Geometry check sheet. Reference: the model listing, model coordinates, mm. A direction names the side the tool comes from. Give positions to 0.01 mm unless a question says otherwise; leave off trailing zeros. Write each loop counter-clockwise with the first axis right and the second up, starting at its lowest first coordinate (ties: lowest second). Pieces come first, ordered by that corner, then holes. Notation, with made-up numbers: (62.25, 7.25) - (102.25, 7.25) arc R10 ccw to (102.25, 25.25) - close; hole circle Ø1 at (51.5, 77). An arc over 180 degrees is marked (long way). Use a Markdown table: item, result.
```python
from build123d import *
from build123d.topology import SkipClean

# Parameters (mm, degrees)
CUT_EXTRUDE_1_REACH             = 16.541
CUT_EXTRUDE_1_DIRECTION_2_DEPTH = 10
PATTERN_CIRCULAR_1_COUNT        = 6
EXTRUDE_1_DEPTH                 = 1
PATTERN_CIRCULAR_2_COUNT        = 4


with BuildPart() as part:
    # Sketch 1 → Revolve 2 (revolve)
    with BuildSketch(Plane.XY, mode=Mode.PRIVATE) as revolve_2_sk:
        Polygon((-1.494617613, 7.636753237), (-8, 1.13137085), (-8.75, 1.13137085), (-8.75, 0.63137085), (-6.2372583, 0.63137085), (-0.363246763, 6.505382387), align=None)
    revolve(revolve_2_sk.sketch.rotate(Axis((0, 35.786073675, 0), (0, -1, 0)), 90), axis=Axis((0, 35.786073675, 0), (0, -1, 0)))

    # Sketch 2 → Cut-Extrude 1 (cut, up to next)
    with BuildSketch(Plane(origin=(0, 0, 0), x_dir=(1, 0, 0), z_dir=(0, 1, 0)), mode=Mode.PRIVATE) as cut_extrude_1_sk1:
        with BuildLine():
            Line((0, -0.1), (7.999374976, -0.1))
            ThreePointArc((7.999374976, -0.1), (8, 0), (7.999374976, 0.1))
            Line((7.999374976, 0.1), (0, 0.1))
            Line((0, 0.1), (0, -0.1))
        make_face()
    cut_extrude_1_tool1 = extrude(cut_extrude_1_sk1.sketch, amount=CUT_EXTRUDE_1_REACH, mode=Mode.PRIVATE) & part.part
    cut_extrude_1 = cut_extrude_1_tool1.solids().sort_by_distance((3.999896, 0, 0))[0]
    add(cut_extrude_1, mode=Mode.SUBTRACT)

    # Sketch 2 → Cut-Extrude 1 direction 2 (cut)
    with BuildSketch(Plane(origin=(0, 0, 0), x_dir=(1, 0, 0), z_dir=(0, 1, 0))):
        with BuildLine():
            Line((0, -0.1), (7.999374976, -0.1))
            ThreePointArc((7.999374976, -0.1), (8, 0), (7.999374976, 0.1))
            Line((7.999374976, 0.1), (0, 0.1))
            Line((0, 0.1), (0, -0.1))
        make_face()
    cut_extrude_1_direction_2 = extrude(amount=-CUT_EXTRUDE_1_DIRECTION_2_DEPTH, mode=Mode.SUBTRACT)

    # Pattern Circular 1: Cut-Extrude 1, Cut-Extrude 1 direction 2 ×6 about axis
    pattern_circular_1_axis = Axis((0, 0, 0), (0, 1, 0))
    add([cut_extrude_1.rotate(pattern_circular_1_axis, i * 360 / PATTERN_CIRCULAR_1_COUNT) for i in range(1, PATTERN_CIRCULAR_1_COUNT)], mode=Mode.SUBTRACT)
    add([cut_extrude_1_direction_2.rotate(pattern_circular_1_axis, i * 360 / PATTERN_CIRCULAR_1_COUNT) for i in range(1, PATTERN_CIRCULAR_1_COUNT)], mode=Mode.SUBTRACT)

    # Sketch 3 → Extrude 1 (add)
    with BuildSketch(Plane(origin=(0, 1.13137085, 0), x_dir=(1, 0, 0), z_dir=(0, 1, 0))):
        with BuildLine():
            Line((-5.366936044, 5.932621469), (-5.897873265, 6.46355869))
            ThreePointArc((-5.897873265, 6.46355869), (-6.187184335, 6.187184335), (-6.46355869, 5.897873265))
            Line((-6.46355869, 5.897873265), (-5.932621469, 5.366936044))
            ThreePointArc((-5.932621469, 5.366936044), (-5.656854249, 5.656854249), (-5.366936044, 5.932621469))
        make_face()
    extrude_1 = extrude(amount=EXTRUDE_1_DEPTH)

    # Pattern Circular 2: Extrude 1 ×4 about axis
    with SkipClean():  # the faces are left unmerged after this step: merging them gives an invalid solid
        pattern_circular_2_axis = Axis((0, 0, 0), (0, 1, 0))
        for i in range(1, PATTERN_CIRCULAR_2_COUNT):
            add(extrude_1.rotate(pattern_circular_2_axis, i * 360 / PATTERN_CIRCULAR_2_COUNT))


solid = part.part
```
1) Section check A-A on y = 5.25. Record the boundary of the cut face in (x, z), then the cut area to 3 significant figures.
Working result:
| item | result |
|---|---|
| outline | (-3.88, -0.1) arc R3.88 ccw to (-2.03, -3.31) - (-0.89, -1.35) arc R1.62 cw to (-1.62, -0.1) - close; (-3.88, 0.1) - (-1.62, 0.1) arc R1.62 cw to (-0.89, 1.35) - (-2.03, 3.31) arc R3.88 ccw to start; (-1.85, -3.41) arc R3.88 ccw to (1.85, -3.41) - (0.72, -1.45) arc R1.62 cw to (-0.72, -1.45) - close; (-1.85, 3.41) - (-0.72, 1.45) arc R1.62 cw to (0.72, 1.45) - (1.85, 3.41) arc R3.88 ccw to start; (0.89, -1.35) - (2.03, -3.31) arc R3.88 ccw to (3.88, -0.1) - (1.62, -0.1) arc R1.62 cw to start; (0.89, 1.35) arc R1.62 cw to (1.62, 0.1) - (3.88, 0.1) arc R3.88 ccw to (2.03, 3.31) - close |
| area | 36.4 mm² |
2) Mould release check, pull along X, two halves, no side actions. Record for faces 6 (the flat face through (2.01, 3.86, -3.68)), 7 (the flat face through (1.99, 3.86, 3.65)), 8 (the flat face through (-6, 2.131, -6)): pulls with the +X half, pulls with the -X half, needs draft (parallel to the pull), parting line crosses it, or undercut.
Working result:
| item | result |
|---|---|
| face 6 | undercut |
| face 7 | undercut |
| face 8 | needs draft |
3) Depth check by flat-ended pin: P1, Ø0.9, axis at x = 6, z = 6, coming from the +Y side; P2, Ø2, axis at x = -3, y = 6, coming from the -Z side; P3, Ø2, axis at x = -2.5, z = -3, coming from the +Y side. Enter the tip coordinate at first touch or a pass-through.
Working result:
| item | result |
|---|---|
| P1 | stops at y = 2.13 |
| P2 | stops at z = -3.12 |
| P3 | stops at y = 6.23 |
4) Section check B-B on z = 4.75. Count the separate pieces of the cut face and the enclosed holes in it, then the cut area to 3 significant figures.
Working result:
| item | result |
|---|---|
| separate pieces | 3 |
| enclosed holes | 0 |
| area | 24.9 mm² |
5) Material ranges on L1, parallel to X at y = 5, z = -2.25; L2, parallel to Z at x = 2, y = 4.5; L3, parallel to X at y = 2, z = -5.5, recorded low to high. Write a range as from..to.
Working result:
| item | result |
|---|---|
| L1 | x = -3.46..-1.41, -1.18..1.18, 1.41..3.46 |
| L2 | z = -4.18..-3.66, -3.26..-1.27, 1.27..3.26, 3.66..4.18 |
| L3 | x = -6.07..-5.81, -4.54..-3.29, -3.06..3.06, 3.29..4.54, 5.81..6.07 |
6) Set-up check for faces 1 (the conical face through (-0.01, 7.08, -0.94)), 2 (the flat face through (-2.01, 3.86, 3.68)), 3 (the flat face through (6, 2.131, 6)), 4 (the flat face through (0, 1.131, 8.2)), 5 (the conical face through (2.83, 3.61, 1.61)): record each of +Z, -Z, +X, -X, +Y, -Y from which the full face is reachable in a straight line by a thin tool's end or side.
Working result:
| item | result |
|---|---|
| face 1 | +Y |
| face 2 | +Y, -Y |
| face 3 | +Z, +X, +Y |
| face 4 | +Z, +Y |
| face 5 | -Y |
